from build123d import *

# Parameters (mm, degrees)
SKETCH1_R           = 5.0038
EXTRUDE1_DEPTH      = 37
SKETCH2_R           = 0.974600032
EXTRUDE2_DEPTH      = 7.5
SKETCH3_OUTSIDE_W   = 19.93
SKETCH3_OUTSIDE_H   = 19.93
SKETCH3_OUTSIDE_R   = 1.5
EXTRUDE3_DEPTH      = 20.32
SKETCH5_R           = 0.635
EXTRUDE4_DEPTH      = 20.32
CHAMFER2_SIZE       = 0.254
SKETCH6_W           = 0.539999936
SKETCH6_H           = 11.68
CHAMFER3_SIZE       = 2.9464
SKETCH8_R           = 4.7498
SKETCH8_R_2         = 0.974600032
BOSS_EXTRUDE1_DEPTH = 1
CHAMFER4_SIZE       = 0.254


with BuildPart() as part:
    # Sketch1 → Extrude1 (new body)
    with BuildSketch(Plane.XY):
        Circle(SKETCH1_R)
    extrude(amount=-EXTRUDE1_DEPTH)

    # Sketch2 → Extrude2 (cut)
    with BuildSketch(Plane.XY):
        Circle(SKETCH2_R)
    extrude(amount=-EXTRUDE2_DEPTH, mode=Mode.SUBTRACT)

    # Sketch3 outside → Extrude3 (cut)
    with BuildSketch(Plane(origin=(0, 0, -37), x_dir=(-1, 0, 0), z_dir=(0, 0, -1))):
        Rectangle(SKETCH3_OUTSIDE_W, SKETCH3_OUTSIDE_H)
        Circle(SKETCH3_OUTSIDE_R, mode=Mode.SUBTRACT)
    extrude(amount=-EXTRUDE3_DEPTH, mode=Mode.SUBTRACT)

    # Sketch5 → Extrude4 (cut)
    with BuildSketch(Plane(origin=(0, 0, 0), x_dir=(0, 0, -1), z_dir=(1, 0, 0))):
        with Locations((7, 0)):
            Circle(SKETCH5_R)
    extrude(amount=-EXTRUDE4_DEPTH, mode=Mode.SUBTRACT)

    # Chamfer2
    chamfer2_edges = [part.edges().sort_by_distance(p)[0] for p in [
        (-5.0038, 0, 0),
    ]]
    chamfer(chamfer2_edges, length=CHAMFER2_SIZE)

    # Sketch6 → Cut-Revolve1 (revolve, cut)
    with BuildSketch(Plane(origin=(0, 0, 0), x_dir=(1, 0, 0), z_dir=(0, 1, 0))):
        with Locations((-4.733800032, 10.84)):
            Rectangle(SKETCH6_W, SKETCH6_H)
    revolve(axis=Axis((0, 0, -37), (0, 0, 1)), mode=Mode.SUBTRACT)

    # Chamfer3
    chamfer3_edges = [part.edges().sort_by_distance(p)[0] for p in [
        (1.5, 0, -16.68),
    ]]
    chamfer(chamfer3_edges, length=CHAMFER3_SIZE)

    # Sketch8 → Boss-Extrude1 (add)
    with BuildSketch(Plane.XY):
        Circle(SKETCH8_R)
        Circle(SKETCH8_R_2, mode=Mode.SUBTRACT)
    extrude(amount=BOSS_EXTRUDE1_DEPTH)

    # Chamfer4
    chamfer4_edges = [part.edges().sort_by_distance(p)[0] for p in [
        (-0.974600032, 0, 1),
    ]]
    chamfer(chamfer4_edges, length=CHAMFER4_SIZE)


solid = part.part
Model file for the job. Use its own axes, mm. A direction names the side the tool comes from. Round coordinates to 2 decimals unless told otherwise and drop trailing zeros. Loops run counter-clockwise (first coordinate to the right, second up) from the corner with the lowest first, then second, coordinate; pieces in that order, holes last. Notation, with made-up numbers: M 7.5,15.25 L 25.5,15.25 A10 ccw 25.5,26.25 Z; hole C 68.5,62 d9. An arc over 180 degrees is marked long. One line per question, with ' | ' between items.
1) Band-saw the part on C-C (z = -29). Give the cut face in (x, y).
Solved:
outline: C 0,0 d3
2) Band-saw the part on B-B (z = -2.5). Give the cut face in (x, y).
Solved:
outline: C 0,0 d10.01; hole C 0,0 d1.95
3) Flat gauge pins, fed straight in: pin 1 (1.5 mm diameter, centred on y = 0, z = -7, fed in from +X); pin 2 (1.5 mm diameter, centred on x = 1.5, z = -12.5, fed in from -Y); pin 3 (1.5 mm diameter, centred on x = -2.5, y = -3.5, fed in from -Z). Where does each tip first touch, or does it go through?
Solved:
pin 1: stops at x = 4.46 | pin 2: stops at y = -4.4 | pin 3: stops at z = -17.58
4) 3-axis set-ups, long thin cutter, end or side, ignore diameter. For faces 4 (the cylindrical face through (-3.5, 3.21, 0.49)), 5 (the cylindrical face through (-2.7, -0.24, -7.59)), 6 (the cylindrical face through (1.5, 0.07, -28.43)): which of +Z, -Z, +X, -X, +Y, -Y reach the whole face in a straight line?
Solved:
face 4: +Z | face 5: -X | face 6: -Z
5) Mould opens along Y. For faces 1 (the flat face through (0.2, 0, -7.5)), 2 (the flat face through (1, -1, 1)), 3 (the conical face through (1.304, -1, -19.483)) say: +Y half, -Y half, draft (parallel to the pull), parting line (faces both ways), or undercut.
Solved:
face 1: undercut | face 2: draft | face 3: parting line
6) Band-saw the part on A-A (y = 0). Give the cut face in (x, z) (3 decimals).
Solved:
outline: M -5.004,-5 L -4.464,-5 L -4.464,-6.365 L -0.975,-6.365 L -0.975,0.746 L -1.229,1 L -4.75,1 L -4.75,0 L -5.004,-0.254 Z; M -4.464,-16.68 L -4.446,-16.68 L -1.5,-19.626 L -1.5,-37 L 1.5,-37 L 1.5,-19.626 L 4.446,-16.68 L 4.464,-16.68 L 4.464,-5 L 5.004,-5 L 5.004,-0.254 L 4.75,0 L 4.75,1 L 1.229,1 L 0.975,0.746 L 0.975,-7.5 L 0,-7.5 L 0,-7.635 L -4.464,-7.635 Z
7) Drill centre lines: line 1 along Y through (x, z) = (0, -3); line 2 along Z through (x, y) = (-0.75, -4.5); line 3 along Z through (x, y) = (-3.75, -0.5). Where is each one in solid material? Low to high.
Solved:
line 1: y = -5 to -0.97, 0.97 to 5 | line 2: z = -5 to 1 | line 3: z = -17.34 to -7.39, -6.61 to 1
8) Band-saw the part on D-D (z = -13.5). Give the cut face in (x, y).
Solved:
outline: C 0,0 d8.93
